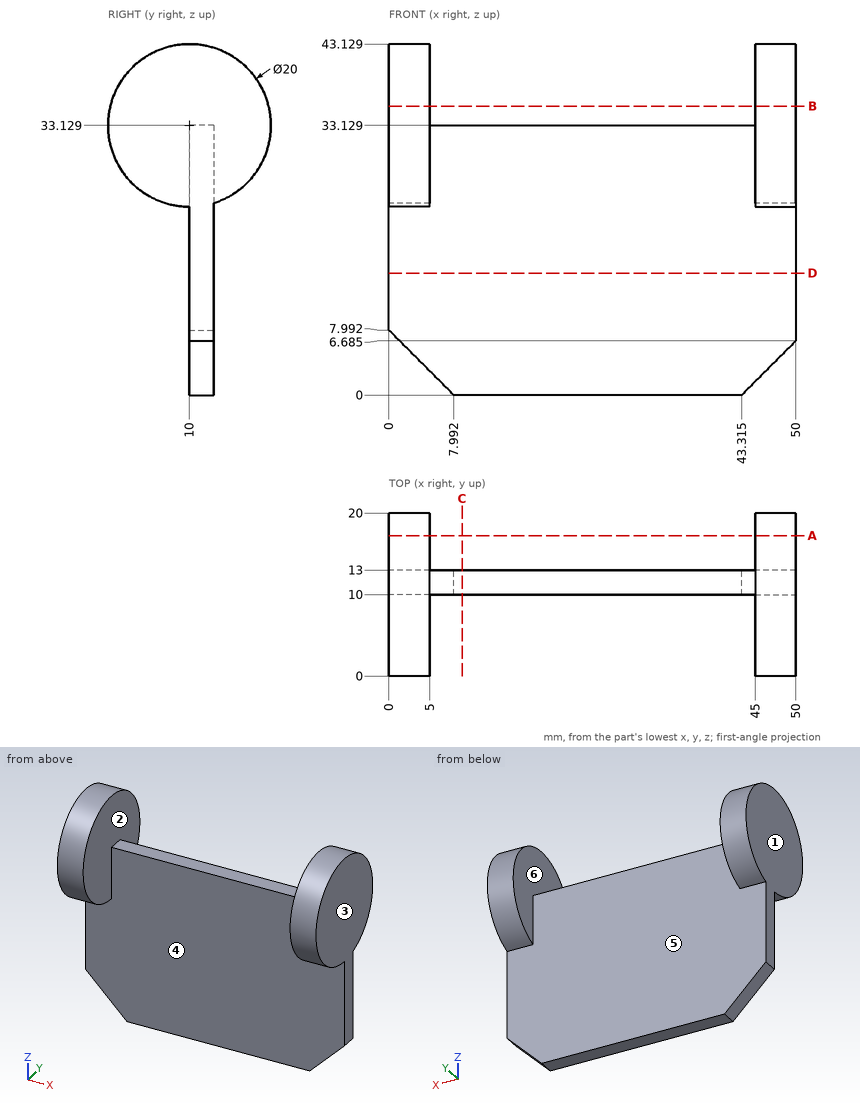
Source: three-view drawing plus pictorial views. Frame: mm from the lowest corner of the part. A direction names the side the tool comes from. Round coordinates to 2 decimals unless told otherwise and drop trailing zeros. Loops run counter-clockwise (first coordinate to the right, second up) from the corner with the lowest first, then second, coordinate; pieces in that order, holes last.
Q1. Pull-direction query (X, two-part tool) for the marked faces 1, 2 and 3; classes: released by +X, released by -X, zero draft, split by the parting line, or undercut.
Q2. Section A-A on y = 17.25. Return loops of the section in (x, z).
Q3. Section C-C on x = 9. Return loops of the section in (y, z).
Q4. Section B-B on z = 35.5. Return loops of the section in (x, y) (1 decimal).
Q5. Pin query (flat end, axial travel): P1, Ø10, axis at x = 26.5, z = 31, coming from the +Y side; P2, Ø2, axis at x = 34, y = 10.5, coming from the +Z side; P3, Ø16.5, axis at x = 31, z = 14.5, coming from the -Y side. Return the tip coordinate at first contact, or that it passes through.
Q6. Material intervals for L1, parallel to X at y = 17.75, z = 36; L2, parallel to Y at x = 33, z = 15; L3, parallel to Z at x = 46.5, y = 17, sorted ascending.
Q7. Section D-D on z = 15. Return loops of the section in (x, y), plus the area to 3 significant figures.
Q8. Access query for the marked faces 4, 5 and 6. Directions: +Z, -Z, +X, -X, +Y, -Y. A direction counts if a zero-diameter tool reaches every point of the face in a straight line with its end or side. Return the directions, or none.
Evaluation:
1. face 1: released by -X
1. face 2: undercut
1. face 3: released by +X
2. outline: (0, 26.24) - (5, 26.24) - (5, 40.02) - (0, 40.02) - close; (45, 26.24) - (50, 26.24) - (50, 40.02) - (45, 40.02) - close
3. outline: (10, 0) - (13, 0) - (13, 33.13) - (10, 33.13) - close
4. outline: (0, 0.3) - (5, 0.3) - (5, 19.7) - (0, 19.7) - close; (45, 0.3) - (50, 0.3) - (50, 19.7) - (45, 19.7) - close
5. P1: stops at y = 13
5. P2: stops at z = 33.13
5. P3: stops at y = 10
6. L1: x = 0 to 5, 45 to 50
6. L2: y = 10 to 13
6. L3: z = 25.99 to 40.27
7. outline: (0, 10) - (50, 10) - (50, 13) - (0, 13) - close
7. area: 150 mm2
8. face 4: -Z, -Y
8. face 5: -Z, +Y
8. face 6: +Z
